```python
from build123d import *

# Parameters (mm, degrees)
AXIAL_HOLES_DEPTH      = 184.274684558
AXIAL_HOLES_DEPTH_BACK = 184.274684558
SKETCH2_R              = 1.65
CUT_EXTRUDE2_START     = 174
SKETCH3_R              = 3
CUT_EXTRUDE2_DEPTH     = 2.7


with BuildPart() as part:
    # Axial profile (mm) → Full revolution (revolve)
    with BuildSketch(Plane.XY, mode=Mode.PRIVATE) as full_revolution_sk:
        Polygon((169.7, 25.6), (174.7, 25.6), (174.7, 24), (176.7, 24), (176.7, 34.4), (169.7, 34.4), align=None)
    revolve(full_revolution_sk.sketch.rotate(Axis((-110, 0, 0), (1, 0, 0)), 90), axis=Axis((-110, 0, 0), (1, 0, 0)))

    # Sketch2 → Axial holes (cut, two sides: drawn at the far end of the back side and taken through both)
    with BuildSketch(Plane(origin=(0, 0, 0), x_dir=(0, 0, -1), z_dir=(1, 0, 0)).offset(-AXIAL_HOLES_DEPTH_BACK)):
        with Locations(Location((29.4, 0, 0), (0, 0, 180))):
            Circle(SKETCH2_R)
        with Locations(Location((-14.7, 25.461146871, 0), (0, 0, 180))):
            Circle(SKETCH2_R)
        with Locations(Location((-14.7, -25.461146871, 0), (0, 0, 180))):
            Circle(SKETCH2_R)
    extrude(amount=AXIAL_HOLES_DEPTH + AXIAL_HOLES_DEPTH_BACK, mode=Mode.SUBTRACT)

    # Sketch3 → Cut-Extrude2 (cut)
    with BuildSketch(Plane(origin=(0, 0, 0), x_dir=(0, 0, -1), z_dir=(1, 0, 0)).offset(CUT_EXTRUDE2_START)):
        with Locations((29.4, 0)):
            Circle(SKETCH3_R)
        with Locations((-14.7, 25.461146871)):
            Circle(SKETCH3_R)
        with Locations((-14.7, -25.461146871)):
            Circle(SKETCH3_R)
    extrude(amount=-CUT_EXTRUDE2_DEPTH, mode=Mode.SUBTRACT)


solid = part.part
```
Geometry: final body of the model. Coordinates: model frame, mm. A direction names the side the tool comes from. Round coordinates to 2 decimals unless told otherwise and drop trailing zeros. Order: outer loops, then holes, each group sorted by start corner. A loop starts at its lowest first (then second) coordinate and runs counter-clockwise, first axis right, second up. Notation, with made-up numbers: (13, 50.5) - (50, 50.5) arc R13 cw to (50, 67.5) - close; hole circle Ø2 at (28.5, 28). An arc over 180 degrees is marked (long way). Write item = value, one per line. Start each with the question number.
Q1. Access query for faces 1 (the flat face through (174.7, -23, -8)), 2 (the cylindrical face through (170.49, 24.07, 15.59)), 3 (the flat face through (171.3, -1, -31)). Directions: +Z, -Z, +X, -X, +Y, -Y. A direction counts if a zero-diameter tool reaches every point of the face in a straight line with its end or side. Return the directions, or none.
Q2. Pin query (flat end, axial travel): pin 1 (1.5 mm diameter, centred on x = 175.5, y = -11, fed in from -Z). Return the tip coordinate at first contact, or that it passes through.
Q3. Cut plane D-D on x = 175.75. Return the cut outline in (y, z).
Q4. Cut plane B-B on z = 0. Return the cut outline in (x, y), and give its area (3 significant figures).
Q5. Cut plane A-A on y = 0. Return the cut outline in (x, z).
Q6. Cut plane C-C on y = -11. Return the cut outline in (x, z).
Q7. Ray query, line 1 (X direction, y = 27.5, z = 15.5); line 2 (Z direction, x = 173, y = -1.5); line 3 (Y direction, x = 175.75, z = 0.5). Return the intervals inside material, ascending. Write a range as from..to.
Q8. Pull-direction query (Z, two-part tool) for faces 4 (the cylindrical face through (170.489, -0.496, -27.826)), 5 (the flat face through (176.7, 7.2, 23.4)); classes: +Z half, -Z half, draft (parallel to the pull), parting line (faces both ways), or undercut.
Outcome:
q1.face_1 = -X
q1.face_2 = +X, -X
q1.face_3 = none
q2.pin_1 = -32.84
q3.outline = circle Ø68.8 at (0, 0); hole circle Ø3.3 at (-25.46, 14.7); hole circle Ø48 at (0, 0); hole circle Ø3.3 at (0, -29.4); hole circle Ø3.3 at (25.46, 14.7)
q4.outline = (169.7, -34.4) - (176.7, -34.4) - (176.7, -24) - (174.7, -24) - (174.7, -25.6) - (169.7, -25.6) - close; (169.7, 25.6) - (174.7, 25.6) - (174.7, 24) - (176.7, 24) - (176.7, 34.4) - (169.7, 34.4) - close
q4.area = 130 mm^2
q5.outline = (169.7, -34.4) - (176.7, -34.4) - (176.7, -31.05) - (174, -31.05) - (174, -32.4) - (171.3, -32.4) - (171.3, -31.05) - (169.7, -31.05) - close; (169.7, -27.75) - (171.3, -27.75) - (171.3, -26.4) - (174, -26.4) - (174, -27.75) - (176.7, -27.75) - (176.7, -24) - (174.7, -24) - (174.7, -25.6) - (169.7, -25.6) - close; (169.7, 25.6) - (174.7, 25.6) - (174.7, 24) - (176.7, 24) - (176.7, 34.4) - (169.7, 34.4) - close
q6.outline = (169.7, -32.59) - (176.7, -32.59) - (176.7, -21.33) - (174.7, -21.33) - (174.7, -23.12) - (169.7, -23.12) - close; (169.7, 23.12) - (174.7, 23.12) - (174.7, 21.33) - (176.7, 21.33) - (176.7, 32.59) - (169.7, 32.59) - close
q7.line_1 = 169.7..171.3, 174..176.7
q7.line_2 = -34.37..-32, -26.8..-25.56, 25.56..34.37
q7.line_3 = -34.4..-23.99, 23.99..34.4
q8.face_4 = undercut
q8.face_5 = draft
